```python
from build123d import *

# Parameters (mm, degrees)
F0_W     = 130.100816
F0_H     = 91.814518
F1_DEPTH = 50
F2_W     = 33.931456
F2_H     = 51.350809
F3_DEPTH = 25
F4_R     = 5


with BuildPart() as f1:
    # F0 (on Top) → F1 (new body)
    with BuildSketch(Plane.XY):
        with Locations((-0.272177, 1.814514)):
            Rectangle(F0_W, F0_H)
    extrude(amount=F1_DEPTH)

    # F2 (on face) → F3 (cut)
    with BuildSketch(Plane.XY.offset(50)):
        with Locations((47.812503, 1.179434)):
            Rectangle(F2_W, F2_H)
    extrude(amount=-F3_DEPTH, mode=Mode.SUBTRACT)

    # F4
    f4_edges = [f1.edges().sort_by_distance(p)[0] for p in [
        (30.846775, 26.854839, 37.5),
        (30.846775, -24.49597, 37.5),
    ]]
    fillet(f4_edges, radius=F4_R)


solid = f1.part
```
Source: CAD feature listing. Evaluate the final solid. Frame: model axes, mm. A direction names the side the tool comes from. Give positions to 0.01 mm unless a question says otherwise; leave off trailing zeros. Write each loop counter-clockwise with the first axis right and the second up, starting at its lowest first coordinate (ties: lowest second). Pieces come first, ordered by that corner, then holes.
1. Section query D-D (y = -22). Return the cut outline in (x, z), then the cut area to 3 significant figures.
2. Section query A-A (y = -1). Return the cut outline in (x, z).
3. Pull-direction query (Y, two-part tool) for faces 3 (the face through (-1, -44.093, 25)), 4 (the face through (-65.323, 1, 25)), 5 (the face through (32.35, 25.43, 37.33)); classes: +Y half, -Y half, draft (parallel to the pull), parting line (faces both ways), or undercut.
4. Section query C-C (x = 47.5). Return the cut outline in (y, z).
5. Section query B-B (z = 43). Return the cut outline in (x, y), then the cut area to 3 significant figures.
6. Access query for faces 1 (the face through (-1, 2, 0)), 2 (the face through (48, 2, 25)). Directions: +Z, -Z, +X, -X, +Y, -Y. A direction counts if a zero-diameter tool reaches every point of the face in a straight line with its end or side. Return the directions, or none.
7. Material intervals for line 1 along Y through (x, z) = (57, 36.5); line 2 along X through (y, z) = (20.5, 46); line 3 along X through (y, z) = (26, 34.5), sorted ascending.
8. First-contact query: pin 1 (7.5 mm diameter, centred on y = 8.5, z = 36, fed in from +X). Flat tip, straight axial feed; report the tip coordinate or a pass-through.
Output values:
1. outline: (-65.32, 0) - (64.78, 0) - (64.78, 25) - (31.52, 25) - (31.52, 50) - (-65.32, 50) - close
1. area: 5,670 mm2
2. outline: (-65.32, 0) - (64.78, 0) - (64.78, 25) - (30.85, 25) - (30.85, 50) - (-65.32, 50) - close
3. face 3: -Y half
3. face 4: draft
3. face 5: undercut
4. outline: (-44.09, 0) - (47.72, 0) - (47.72, 50) - (26.85, 50) - (26.85, 25) - (-24.5, 25) - (-24.5, 50) - (-44.09, 50) - close
5. outline: (-65.32, -44.09) - (64.78, -44.09) - (64.78, -24.5) - (35.85, -24.5) arc R5 cw to (30.85, -19.5) - (30.85, 21.85) arc R5 cw to (35.85, 26.85) - (64.78, 26.85) - (64.78, 47.72) - (-65.32, 47.72) - close
5. area: 10,200 mm2
6. face 1: -Z, +X, -X, +Y, -Y
6. face 2: +Z, +X
7. line 1: y = -44.09 to -24.5, 26.85 to 47.72
7. line 2: x = -65.32 to 30.85
7. line 3: x = -65.32 to 33.05
8. pin 1: stops at x = 30.85
